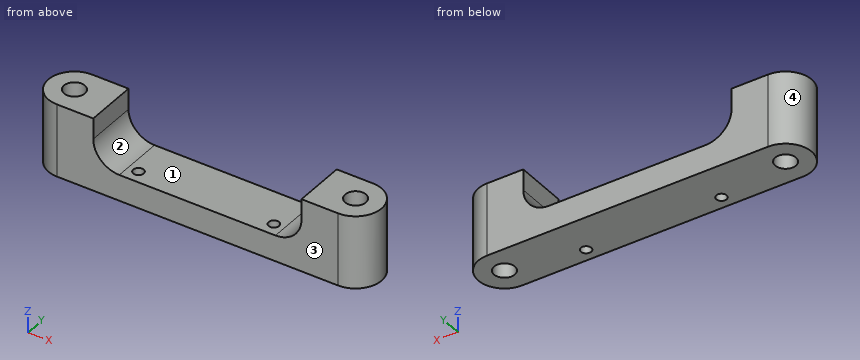
```python
from build123d import *

# Parameters (mm, degrees)
SKETCH_R     = 2
SKETCH_R_2   = 1
PAD_DEPTH    = 14
POCKET_DEPTH = 82.664608


with BuildPart() as part:
    # Sketch → Pad (new body)
    with BuildSketch(Plane.XY):
        with BuildLine():
            ThreePointArc((-26.999971, 5), (-32, 0), (-26.999971, -5))
            Line((-26.999971, -5), (0, -5))
            Line((0, -5), (0, 5))
            Line((-26.999971, 5), (0, 5))
        make_face()
        with Locations((-27, 0)):
            Circle(SKETCH_R, mode=Mode.SUBTRACT)
        with Locations((-13, -2.5)):
            Circle(SKETCH_R_2, mode=Mode.SUBTRACT)
    pad = extrude(amount=PAD_DEPTH)

    # Sketch001 → Pocket (cut, through all)
    with BuildSketch(Plane.XZ.offset(5)):
        with BuildLine():
            Line((-20, 14), (-20, 10.000019))
            ThreePointArc((-20, 10.000019), (-18.535534, 6.464466), (-14.999981, 5))
            Line((0, 5), (-14.999981, 5))
            Line((0, 14), (0, 5))
            Line((-20, 14), (0, 14))
        make_face()
    pocket = extrude(amount=-POCKET_DEPTH, mode=Mode.SUBTRACT)

    # Mirrored: Pad, Pocket across Sketch001 V_Axis
    add(pad.mirror(Plane(origin=(0, -5, 0), x_dir=(0, -1, 0), z_dir=(1, 0, 0))))
    add(pocket.mirror(Plane(origin=(0, -5, 0), x_dir=(0, -1, 0), z_dir=(1, 0, 0))), mode=Mode.SUBTRACT)


solid = part.part
```
Can you work these out from the model? Positions are in its coordinate system, mm. Face numbers are marked on the shaded views. Coordinates: 2 decimals unless noted, no trailing zeros. Loops run counter-clockwise (first coordinate to the right, second up) from the corner with the lowest first, then second, coordinate; pieces in that order, holes last. Notation, with made-up numbers: (40.5, 41) - (44.5, 41) arc R13 ccw to (44.5, 57) - close; hole circle Ø3 at (40.25, 55). An arc over 180 degrees is marked (long way). Answer as CSV lines item,"result". Start each with the question number.
1) Suppose I cut it at D-D (z = 7.5). Please give me the cut outline in (x, y).
2) Suppose I cut it at B-B (x = -13). Please give me the cut outline in (y, z).
3) For pin 1 (2 mm diameter, centred on y = 1.5, z = 1.5, fed in from +X); pin 2 (2.5 mm diameter, centred on x = 27, y = 0, fed in from -Z); pin 3 (3 mm diameter, centred on x = 5.5, y = -1.5, fed in from +Z); pin 4 (1 mm diameter, centred on y = 2.5, z = 8, fed in from +X), each with a flat end and sliding along its axis, tell me the tip position at first contact or that it passes through.
4) Thinking about a two-plate mould opening in X: for the marked faces 1, 2, 3 and 4, which applies, pulls with the +X half, pulls with the -X half, needs draft (parallel to the pull), parting line crosses it, or undercut?
5) Suppose I cut it at A-A (z = 11). Please give me the cut outline in (x, y), plus the area to 3 significant figures.
6) I need wall thicknesses on line 1 (Y direction, x = 27, z = 9.75); line 2 (X direction, y = 1.5, z = 12.75); line 3 (X direction, y = 0.25, z = 0.5). Which ranges of each line are inside material? Lowest first, please. Write a range as from..to.
7) Suppose I cut it at C-C (y = 0). Please give me the cut outline in (x, z).
Check result:
1,outline,"(-27, -5) - (-19.33, -5) - (-19.33, 5) - (-27, 5) arc R5 ccw to start; (19.33, -5) - (27, -5) arc R5 ccw to (27, 5) - (19.33, 5) - close; hole circle Ø4 at (-27, 0); hole circle Ø4 at (27, 0)"
2,outline,"(-5, 0) - (-3.5, 0) - (-3.5, 5) - (-5, 5) - close; (-1.5, 0) - (5, 0) - (5, 5) - (-1.5, 5) - close"
3,pin 1,"stops at x = 31.97"
3,pin 2,"passes through"
3,pin 3,"stops at z = 5"
3,pin 4,"stops at x = 31.58"
4,face 1,"undercut"
4,face 2,"undercut"
4,face 3,"needs draft"
4,face 4,"pulls with the -X half"
5,outline,"(-27, -5) - (-20, -5) - (-20, 5) - (-27, 5) arc R5 ccw to start; (20, -5) - (27, -5) arc R5 ccw to (27, 5) - (20, 5) - close; hole circle Ø4 at (-27, 0); hole circle Ø4 at (27, 0)"
5,area,"193 mm²"
6,line 1,"y = -5..-2, 2..5"
6,line 2,"x = -31.77..-28.32, -25.68..-20, 20..25.68, 28.32..31.77"
6,line 3,"x = -31.99..-28.98, -25.02..25.02, 28.98..31.99"
7,outline,"(-32, 0) - (-29, 0) - (-29, 14) - (-32, 14) - close; (-25, 0) - (25, 0) - (25, 14) - (20, 14) - (20, 10) arc R5 cw to (15, 5) - (-15, 5) arc R5 cw to (-20, 10) - (-20, 14) - (-25, 14) - close; (29, 0) - (32, 0) - (32, 14) - (29, 14) - close"
